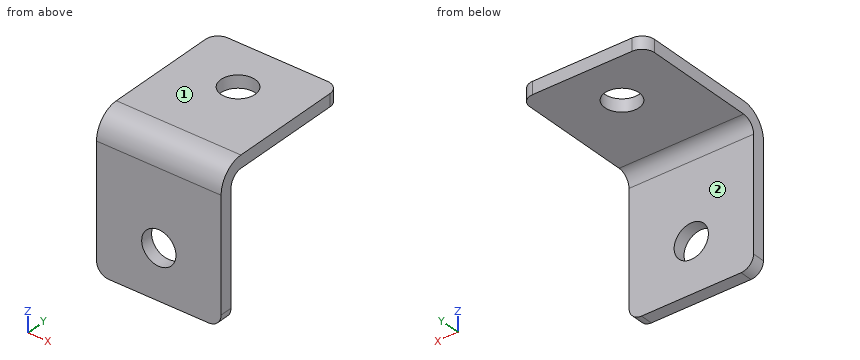
from build123d import *

# Parameters (mm, degrees)
BASE_FLANGE1_DEPTH = 31.75
SKETCH6_R          = 4.3688
CUT_EXTRUDE1_DEPTH = 63.540247041
SKETCH7_R          = 4.3688
CUT_EXTRUDE2_DEPTH = 63.540247041
FILLET1_R          = 3.175


# Sheet-metal steps are written as plain solids
with BuildPart() as part:
    # Sketch1 → Base-Flange1 (new body)
    with BuildSketch(Plane(origin=(0, 0, 0), x_dir=(0, 0, -1), z_dir=(1, 0, 0))):
        with BuildLine():
            Line((38.1, 0), (6.35, 0))
            ThreePointArc((6.35, 0), (1.859871939, 1.859871939), (0, 6.35))
            Line((0, 6.35), (0, 38.1))
            Line((0, 38.1), (3.175, 38.1))
            Line((3.175, 38.1), (3.175, 6.35))
            ThreePointArc((3.175, 6.35), (4.10493597, 4.10493597), (6.35, 3.175))
            Line((6.35, 3.175), (38.1, 3.175))
            Line((38.1, 3.175), (38.1, 0))
        make_face()
    extrude(amount=BASE_FLANGE1_DEPTH)

    # Sketch6 → Cut-Extrude1 (cut, through all)
    with BuildSketch(Plane.XY):
        with Locations((15.875, 25.4)):
            Circle(SKETCH6_R)
    extrude(amount=-CUT_EXTRUDE1_DEPTH, mode=Mode.SUBTRACT)

    # Sketch7 → Cut-Extrude2 (cut, through all)
    with BuildSketch(Plane.XZ):
        with Locations(Location((15.875, -25.4, 0), (0, 0, 270))):
            Circle(SKETCH7_R)
    extrude(amount=-CUT_EXTRUDE2_DEPTH, mode=Mode.SUBTRACT)

    # Fillet1
    fillet1_edges = [part.edges().sort_by_distance(p)[0] for p in [
        (31.75, 38.1, -1.5875),
        (0, 38.1, -1.5875),
        (31.75, 1.5875, -38.1),
        (0, 1.5875, -38.1),
    ]]
    fillet(fillet1_edges, radius=FILLET1_R)


solid = part.part
Part model, mm, in its own coordinate system. Face numbers are marked on the shaded views. A direction names the side the tool comes from. Give positions to 0.01 mm unless a question says otherwise; leave off trailing zeros. Loops run counter-clockwise (first coordinate to the right, second up) from the corner with the lowest first, then second, coordinate; pieces in that order, holes last.
(1) Band-saw the part on D-D (x = 21). Write the cut outline in (y, z) (3 decimals), and give its area (3 significant figures).
Return value:
outline: (0, -38.1) - (3.175, -38.1) - (3.175, -6.35) arc R3.175 cw to (6.35, -3.175) - (38.1, -3.175) - (38.1, 0) - (6.35, 0) arc R6.35 ccw to (0, -6.35) - close
area: 225 mm2
(2) Band-saw the part on A-A (z = -25.4). Write the cut outline in (x, y) (3 decimals).
Return value:
outline: (0, 0) - (11.506, 0) - (11.506, 3.175) - (0, 3.175) - close; (20.244, 0) - (31.75, 0) - (31.75, 3.175) - (20.244, 3.175) - close
(3) Band-saw the part on C-C (x = 14.5). Write the cut outline in (y, z) (3 decimals).
Return value:
outline: (0, -38.1) - (3.175, -38.1) - (3.175, -29.547) - (0, -29.547) - close; (0, -21.253) - (3.175, -21.253) - (3.175, -6.35) arc R3.175 cw to (6.35, -3.175) - (21.253, -3.175) - (21.253, 0) - (6.35, 0) arc R6.35 ccw to (0, -6.35) - close; (29.547, -3.175) - (38.1, -3.175) - (38.1, 0) - (29.547, 0) - close
(4) Drill centre lines: line 1 along X through (y, z) = (2.4, -25.4); line 2 along Z through (x, y) = (18, 10) (3 decimals); line 3 along Y through (x, z) = (19.5, -16) (3 decimals). Where is each one in solid material? Low to high.
Return value:
line 1: x = 0 to 11.51, 20.24 to 31.75
line 2: z = -3.175 to 0
line 3: y = 0 to 3.175
(5) 3-axis set-ups, long thin cutter, end or side, ignore diameter. For the marked faces 1 and 2: which of +Z, -Z, +X, -X, +Y, -Y reach the whole face in a straight line?
Return value:
face 1: +Z, +X, -X, +Y, -Y
face 2: -Z, +X, -X, +Y
(6) Pin check, flat tips, straight feed: pin 1 (6 mm diameter, centred on y = 15.5, z = -4.5, fed in from -X); pin 2 (16 mm diameter, centred on x = 12, y = 16, fed in from -Z) (3 decimals); pin 3 (4 mm diameter, centred on x = 16, z = -5.5, fed in from +Y). Stop position of each tip, or through.
Return value:
pin 1: stops at x = 0
pin 2: stops at z = -3.175
pin 3: stops at y = 4.95
(7) Band-saw the part on B-B (y = 25.4). Write the cut outline in (x, z) (3 decimals), and give its area (3 significant figures).
Return value:
outline: (0, -3.175) - (11.506, -3.175) - (11.506, 0) - (0, 0) - close; (20.244, -3.175) - (31.75, -3.175) - (31.75, 0) - (20.244, 0) - close
area: 73.1 mm2
